Design review of the part built by this model. Coordinates are the model's own, in mm. A direction names the side the tool comes from. Round coordinates to 2 decimals unless told otherwise and drop trailing zeros. Loops run counter-clockwise (first coordinate to the right, second up) from the corner with the lowest first, then second, coordinate; pieces in that order, holes last. Notation, with made-up numbers: (41.5, 30) - (80.5, 30) arc R19 ccw to (80.5, 64) - close; hole circle Ø3 at (78, 42.25). An arc over 180 degrees is marked (long way). Use one line per item in the form item = value. Start each with the question number.
(1) The part is to be moulded in two halves that separate along Y. For faces 3 (the cylindrical face through (5.84, -7.11, 0.25)), 4 (the cylindrical face through (8.54, -6.773, 0.246)), 5 (the flat face through (0, -10, 0)), say which applies: released by +Y, released by -Y, zero draft, split by the parting line, or undercut.
(2) Machinability: for faces 1 (the cylindrical face through (0.1, -9.3, 0.2)), 2 (the cylindrical face through (-5.82, -7.125, 0.246)), which of the approach directions +Z, -Z, +X, -X, +Y, -Y give a long, thin tool a straight path to every point of the face, cutting with its end or side? Answer none if there is none.
(3) We need section D-D, the plane x = -3.75. Write out the cut boundary in (y, z).
(4) We need section C-C, the plane y = -8.5. Write out the cut boundary in (x, z).
(5) Wall thickness on probe 1 along Y at (x, z) = (0.25, 0.35); probe 2 along X at (y, z) = (-7.5, 0.25); probe 3 along X at (y, z) = (-6, 0.4): over which ranges is each line inside the solid? List them lowest first. Write a range as [from, to].
(6) We need section B-B, the plane z = 0.25. Write out the cut boundary in (x, y).
(7) We need section A-A, the plane y = -6.25. Write out the cut boundary in (x, z), then the cut area to 3 significant figures.
from build123d import *

# Parameters (mm, degrees)
OTHER_10076_5_DEPTH = 0.5
CUT_EXTRUDE1_START  = -0.5
CUT_EXTRUDE1_DEPTH  = 0.5


# Read off the part's stored shape, not the designer's step: 10076-5
with BuildPart() as part:
    # Other 10076-5 outline → Other 10076-5 (new body)
    with BuildSketch(Plane.XY):
        with BuildLine():
            ThreePointArc((7.573674013, -9.436602245), (7.668819519, -9.359444812), (7.763179028, -9.281328104))
            Line((7.763179028, -9.281328104), (7.919995926, -7.488902759))
            ThreePointArc((7.919995926, -7.488902759), (8.548470738, -6.76266575), (9.110578105, -5.983925684))
            ThreePointArc((9.110578105, -5.983925684), (9.242448569, -5.182849851), (8.736493865, -4.547930843))
            Line((8.736493865, -4.547930843), (8.260223146, -4.3))
            Line((8.260223146, -4.3), (5.774945887, -4.3))
            ThreePointArc((5.774945887, -4.3), (5.659072475, -4.451392897), (5.53923133, -4.5996648))
            Line((5.53923133, -4.5996648), (6.59, -6.419649523))
            ThreePointArc((6.59, -6.419649523), (5.831509763, -7.1157216), (5, -7.722693831))
            Line((5, -7.722693831), (5, -7.841555968))
            ThreePointArc((5, -7.841555968), (0, -9.3), (-5, -7.841555968))
            Line((-5, -7.841555968), (-5, -7.722693831))
            ThreePointArc((-5, -7.722693831), (-5.831509763, -7.1157216), (-6.59, -6.419649523))
            Line((-6.59, -6.419649523), (-5.53923133, -4.5996648))
            ThreePointArc((-5.53923133, -4.5996648), (-5.659072475, -4.451392897), (-5.774945887, -4.3))
            Line((-5.774945887, -4.3), (-8.260223146, -4.3))
            Line((-8.260223146, -4.3), (-10.732831081, -5.58715822))
            ThreePointArc((-10.732831081, -5.58715822), (-10.675718173, -5.6955282), (-10.617511084, -5.803314431))
            Line((-10.617511084, -5.803314431), (-9.055174855, -6.258693914))
            ThreePointArc((-9.055174855, -6.258693914), (-8.704696722, -6.64117368), (-8.882127626, -7.128661083))
            Line((-8.882127626, -7.128661083), (-9.436602245, -7.573674013))
            ThreePointArc((-9.436602245, -7.573674013), (-9.359444812, -7.668819519), (-9.281328104, -7.763179028))
            Line((-9.281328104, -7.763179028), (-7.660171598, -7.905011844))
            ThreePointArc((-7.660171598, -7.905011844), (-7.241809703, -8.211767477), (-7.320727248, -8.724502998))
            Line((-7.320727248, -8.724502998), (-7.777730077, -9.269137762))
            ThreePointArc((-7.777730077, -9.269137762), (-7.683493234, -9.347402405), (-7.588468891, -9.424709008))
            Line((-7.588468891, -9.424709008), (-5.970792243, -9.247544602))
            ThreePointArc((-5.970792243, -9.247544602), (-5.500623999, -9.466787654), (-5.477995427, -9.985067155))
            Line((-5.477995427, -9.985067155), (-5.819964104, -10.608393744))
            ThreePointArc((-5.819964104, -10.608393744), (-5.712269322, -10.666769858), (-5.603989074, -10.724052707))
            Line((-5.603989074, -10.724052707), (-4.05195869, -10.234699407))
            ThreePointArc((-4.05195869, -10.234699407), (-3.548052399, -10.358004491), (-3.424747314, -10.861910782))
            Line((-3.424747314, -10.861910782), (-3.638540174, -11.539975104))
            ThreePointArc((-3.638540174, -11.539975104), (-3.521526102, -11.576219327), (-3.404151099, -11.611277074))
            Line((-3.404151099, -11.611277074), (-1.977410637, -10.828540453))
            ThreePointArc((-1.977410637, -10.828540453), (-1.459131136, -10.851169025), (-1.239888083, -11.321337268))
            Line((-1.239888083, -11.321337268), (-1.317289186, -12.028081692))
            ThreePointArc((-1.317289186, -12.028081692), (-1.195452609, -12.04080118), (-1.073493507, -12.052286575))
            Line((-1.073493507, -12.052286575), (0.173128198, -11.006246762))
            ThreePointArc((0.173128198, -11.006246762), (0.685863719, -10.927329218), (0.992619352, -11.345691113))
            Line((0.992619352, -11.345691113), (1.054584487, -12.053955847))
            ThreePointArc((1.054584487, -12.053955847), (1.176561457, -12.042661796), (1.298417839, -12.030133462))
            Line((1.298417839, -12.030133462), (2.317013814, -10.760989181))
            ThreePointArc((2.317013814, -10.760989181), (2.804501216, -10.583558277), (3.186980982, -10.93403641))
            Line((3.186980982, -10.93403641), (3.38593107, -11.616603238))
            ThreePointArc((3.38593107, -11.616603238), (3.503360927, -11.581729673), (3.620431715, -11.545669067))
            Line((3.620431715, -11.545669067), (4.371857887, -10.10219282))
            ThreePointArc((4.371857887, -10.10219282), (4.815363304, -9.833067127), (5.258868721, -10.10219282))
            Line((5.258868721, -10.10219282), (5.58715822, -10.732831081))
            ThreePointArc((5.58715822, -10.732831081), (5.6955282, -10.675718173), (5.803314431, -10.617511084))
            Line((5.803314431, -10.617511084), (6.258693914, -9.055174855))
            ThreePointArc((6.258693914, -9.055174855), (6.64117368, -8.704696722), (7.128661083, -8.882127626))
            Line((7.128661083, -8.882127626), (7.573674013, -9.436602245))
        make_face()
    extrude(amount=OTHER_10076_5_DEPTH)

    # Sketch1 → Cut-Extrude1 (cut)
    with BuildSketch(Plane.XY.offset(0.5).offset(CUT_EXTRUDE1_START)):
        with BuildLine():
            Line((-9.668418082, -5.033059884), (-10.732831081, -5.58715822))
            ThreePointArc((-10.732831081, -5.58715822), (-3.521526102, -11.576219327), (5.803314431, -10.617511084))
            Line((5.803314431, -10.617511084), (6.258693914, -9.055174855))
            ThreePointArc((6.258693914, -9.055174855), (6.329177308, -8.908251896), (6.443160998, -8.791795969))
            ThreePointArc((6.443160998, -8.791795969), (-2.476407691, -10.614961373), (-9.668418082, -5.033059884))
        make_face()
    extrude(amount=CUT_EXTRUDE1_DEPTH, mode=Mode.SUBTRACT)


solid = part.part
Data:
q1.face_3 = undercut
q1.face_4 = released by -Y
q1.face_5 = zero draft
q2.face_1 = +Z, -Z, +Y
q2.face_2 = +Z, -Z
q3.outline = (-10.23, 0) - (-8.51, 0) - (-8.51, 0.5) - (-10.23, 0.5) - close
q4.outline = (-6.82, 0) - (-3.77, 0) - (-3.77, 0.5) - (-6.82, 0.5) - close; (3.77, 0) - (7.83, 0) - (7.83, 0.5) - (3.77, 0.5) - close
q5.probe_1 = [-10.9, -9.3]
q5.probe_2 = [-7.91, -5.33], [5.33, 7.92]
q5.probe_3 = [-9.1, -6.35], [6.35, 9.1]
q6.outline = (-9.67, -5.03) arc R10.9 ccw to (6.44, -8.79) arc R0.5 cw to (7.13, -8.88) - (7.57, -9.44) arc R12.1 ccw to (7.76, -9.28) - (7.92, -7.49) arc R10.9 ccw to (9.11, -5.98) arc R1 ccw to (8.74, -4.55) - (8.26, -4.3) - (5.77, -4.3) arc R7.2 cw to (5.54, -4.6) - (6.59, -6.42) arc R9.2 cw to (5, -7.72) - (5, -7.84) arc R9.3 cw to (-5, -7.84) - (-5, -7.72) arc R9.2 cw to (-6.59, -6.42) - (-5.54, -4.6) arc R7.2 cw to (-5.77, -4.3) - (-8.26, -4.3) - close
q7.outline = (-8.93, 0) - (-6.49, 0) - (-6.49, 0.5) - (-8.93, 0.5) - close; (6.49, 0) - (8.93, 0) - (8.93, 0.5) - (6.49, 0.5) - close
q7.area = 2.44 mm^2
